Autodesk Inventor part; units mm, degrees
ref_plane "YZ Plane" through (0, 0, 0) normal (1, 0, 0) x (0, 1, 0)
ref_plane "XZ Plane" through (0, 0, 0) normal (0, 1, 0) x (-1, 0, 0)
ref_plane "XY Plane" through (0, 0, 0) normal (0, 0, 1) x (1, 0, 0)
sketch "Эскиз1" plane through (0, 0, 0) normal (0, 0, 1) x (1, 0, 0)
  line L0 (-2.03, 1.5) -> (2.03, 1.5)
  line L1 (2.03, 1.5) -> (2.03, -1.5)
  line L2 (2.03, -1.5) -> (-2.03, -1.5)
  line L3 (-2.03, -1.5) -> (-2.03, 1.5)
  line L4 (-2.03, 1.5) -> (2.03, -1.5) construction
  line L5 (2.03, 1.5) -> (-2.03, -1.5) construction
  line L6 (-1.6, -1.5) -> (1.6, -1.5)
  line L7 (1.6, -1.5) -> (1.6, -16.5)
  line L8 (1.6, -16.5) -> (-1.6, -16.5)
  line L9 (-1.6, -16.5) -> (-1.6, -1.5)
  line L10 (0, 4.8) -> (0, -22.5041) construction
  line L11 (-7, 4.8) -> (-7, -22.5041)
  line L12 (7, -22.5041) -> (7, 4.8)
  arc A0 (7, 4.8) -> (-7, 4.8) centre (0, 4.8) ccw
  arc A1 (-7, -22.5041) -> (7, -22.5041) centre (0, -22.5041) ccw
  line L13 (-1.6, -1.5) -> (-1.6, -9)
  line L14 (1.6, -1.5) -> (1.6, -9)
  line L15 (-1.6, -5.25) -> (-5.6947, -16.5)
  line L16 (1.6, -5.25) -> (5.6947, -16.5)
  arc A2 (-5.6947, -16.5) -> (5.6947, -16.5) centre (0, -0.854) ccw
  line L17 (1.6, -5.25) -> (-1.6, -5.25)
  circle A3 centre (0, -25.0041) radius 1.5
  circle A4 centre (0, 7.3) radius 1.5
  point P0 (0, 0)
  point P1 (0, 0)
  point P2 (0, 0)
  point P3 (0, 0)
  point P4 (0, -1.5)
  point P5 (0, 0)
  point P6 (0, -8.8521)
  point P7 (1.6, -5.25)
  point P8 (-1.6, -5.25)
  point P9 (1.6, -1.5)
  dimension "d0" = 4.06
  dimension "d1" = 3
  dimension "d2" = 3.2
  dimension "d3" = 15
  dimension "d4" = 14
  dimension "d5" = 20
  dimension "d6" = 20
  dimension "d15" = 3
  dimension "d16" = 3
  dimension "d17" = 3
  dimension "d18" = 3
  dimension "d20" = 6
  dimension "d24" = 16.1521
extrude "Выдавливание1" add sketch "Эскиз1" along normal blind 2 and the other way blind 6.5 contours L0 L1 L2 L3 | L2 L7 L17 L9 | L17 L7 L8 L9 | L9 L8 L7 L16 A2 L15 | A0 L12 A1 L11
extrude "Выдавливание2" cut sketch "Эскиз1" along normal up to surface (2 mm away) draft 60 contours L17 L7 L8 L9
extrude "Выдавливание3" cut sketch "Эскиз1" along normal up to surface (2 mm away) contours L0 L1 L2 L3 | L2 L7 L17 L9
sketch "Эскиз2" plane through (0, 0, 2) normal (0, 0, 1) x (1, 0, 0)
  circle A0 centre (0, 7.3) radius 1.5
  circle A1 centre (0, -25.0041) radius 1.5
  circle A2 centre (0, 7.3) radius 3
  circle A3 centre (0, -25.0041) radius 3
  point P0 (0, 0)
  dimension "d21" = 6
extrude "Выдавливание4" cut sketch "Эскиз2" against normal blind 5.5 contours A0 | A1 | A2 | A3
properties part number "Установка датчика холла"
CAD build for the part. Positions are in the model's coordinates, mm. A direction names the side the tool comes from. Coordinates: 2 decimals unless noted, no trailing zeros. Loops run counter-clockwise (first coordinate to the right, second up) from the corner with the lowest first, then second, coordinate; pieces in that order, holes last. Notation, with made-up numbers: (-0.5, 70) - (3.5, 70) arc R7 ccw to (3.5, 80) - close; hole circle Ø11 at (39.25, 8.5). An arc over 180 degrees is marked (long way). Return JSON: item names as keys, results as strings.
1. Mould opens along X. For faces 3 (the cylindrical face through (-0.39, -22.03, -0.71)), 4 (the flat face through (-7, -9, -2)), 5 (the flat face through (0, -9, -6.5)) say: released by +X, released by -X, zero draft, split by the parting line, or undercut.
Result:
{"face 3": "undercut", "face 4": "released by -X", "face 5": "zero draft"}
2. Band-saw the part on A-A (x = 0). Give the cut face in (y, z).
Result:
{"outline": "(-29.5, -6.5) - (-26.5, -6.5) - (-26.5, -3.5) - (-28, -3.5) - (-28, 2) - (-29.5, 2) - close; (-23.5, -6.5) - (5.8, -6.5) - (5.8, -3.5) - (4.3, -3.5) - (4.3, 2) - (1.5, 2) - (1.5, 0) - (-16.5, 0) - (-19.96, 2) - (-22, 2) - (-22, -3.5) - (-23.5, -3.5) - close; (8.8, -6.5) - (11.8, -6.5) - (11.8, 2) - (10.3, 2) - (10.3, -3.5) - (8.8, -3.5) - close"}
3. 3-axis set-ups, long thin cutter, end or side, ignore diameter. For faces 1 (the cylindrical face through (-0.2, -29.5, -2.2)), 2 (the flat face through (1.6, -3, 1)): which of +Z, -Z, +X, -X, +Y, -Y reach the whole face in a straight line?
Result:
{"face 1": "+Z, -Z, -Y", "face 2": "+Z"}
4. Band-saw the part on C-C (z = -0.75). Give the cut face in (x, y).
Result:
{"outline": "(-7, -22.5) arc R7 ccw to (7, -22.5) - (7, 4.8) arc R7 ccw to (-7, 4.8) - close; hole circle Ø6 at (0, -25); hole circle Ø6 at (0, 7.3)"}
5. Band-saw the part on D-D (y = -16). Give the cut face in (x, z), and give its area (3 significant figures).
Result:
{"outline": "(-7, -6.5) - (7, -6.5) - (7, 2) - (5.06, 2) - (1.6, 0) - (-1.6, 0) - (-5.06, 2) - (-7, 2) - close", "area": "106 mm2"}
6. Drop flat-ended pins along their axis: pin 1 (3 mm diameter, centred on x = -0.5, y = -7.5, fed in from +Z); pin 2 (2.5 mm diameter, centred on x = 0, y = -25, fed in from -Z); pin 3 (1.5 mm diameter, centred on x = -3.5, z = -1.5, fed in from +Y); pin 4 (3 mm diameter, centred on x = -2, z = -2, fed in from +Y). Give the stop position or say it passes through.
Result:
{"pin 1": "stops at z = 0.23", "pin 2": "passes through", "pin 3": "stops at y = 11.24", "pin 4": "stops at y = 11.78"}
7. Probe L1, parallel to Y at x = 0, z = -4.75; L2, parallel to Y at x = 0, z = -1.5; L3, parallel to Y at x = -5.75, z = -1.5. List the from-to ranges inside material, lowest first. Write a range as from..to.
Result:
{"L1": "y = -29.5..-26.5, -23.5..5.8, 8.8..11.8", "L2": "y = -29.5..-28, -22..4.3, 10.3..11.8", "L3": "y = -26.5..8.79"}
8. Band-saw the part on B-B (y = 8). Give the cut face in (x, z), and give its area (3 significant figures).
Result:
{"outline": "(-6.23, -6.5) - (-1.33, -6.5) - (-1.33, -3.5) - (-2.92, -3.5) - (-2.92, 2) - (-6.23, 2) - close; (1.33, -6.5) - (6.23, -6.5) - (6.23, 2) - (2.92, 2) - (2.92, -3.5) - (1.33, -3.5) - close", "area": "65.8 mm2"}
